Work out the finished part from the listing and answer in its coordinate system (mm). Face numbers are marked on the shaded views. A direction names the side the tool comes from. Give positions to 0.01 mm unless a question says otherwise; leave off trailing zeros. Loops run counter-clockwise (first coordinate to the right, second up) from the corner with the lowest first, then second, coordinate; pieces in that order, holes last. Notation, with made-up numbers: M 32,70.25 L 61,70.25 A21 ccw 61,80.25 Z; hole C 45,9 d1. An arc over 180 degrees is marked long. Use a Markdown table: item, result.
```python
from build123d import *

# Parameters (mm, degrees)
F1_DEPTH = 100
F2_R     = 40
F3_DEPTH = 25
F4_R     = 5
F5_DEPTH = 50


with BuildPart() as f1:
    # F0 (on Front) → F1 (new body)
    with BuildSketch(Plane.XZ):
        with BuildLine():
            Line((-58.053203, 88.663405), (-160.553203, 88.663405))
            ThreePointArc((-160.553203, 88.663405), (-164.088737, 87.198939), (-165.553203, 83.663405))
            Line((-165.553203, 83.663405), (-165.553203, -56.336595))
            ThreePointArc((-165.553203, -56.336595), (-164.088737, -59.872129), (-160.553203, -61.336595))
            Line((-160.553203, -61.336595), (129.446797, -61.336595))
            ThreePointArc((129.446797, -61.336595), (132.98233, -59.872129), (134.446797, -56.336595))
            Line((134.446797, -56.336595), (134.446797, 83.663405))
            ThreePointArc((134.446797, 83.663405), (132.98233, 87.198939), (129.446797, 88.663405))
            Line((129.446797, 88.663405), (26.946797, 88.663405))
            ThreePointArc((26.946797, 88.663405), (23.411263, 87.198939), (21.946797, 83.663405))
            Line((21.946797, 83.663405), (21.946797, 43.663405))
            ThreePointArc((21.946797, 43.663405), (20.48233, 40.127871), (16.946797, 38.663405))
            Line((16.946797, 38.663405), (-48.053203, 38.663405))
            ThreePointArc((-48.053203, 38.663405), (-51.588737, 40.127871), (-53.053203, 43.663405))
            Line((-53.053203, 43.663405), (-53.053203, 83.663405))
            ThreePointArc((-53.053203, 83.663405), (-54.51767, 87.198939), (-58.053203, 88.663405))
        make_face()
    extrude(amount=F1_DEPTH)

    # F2 (on face) → F3 (cut)
    with BuildSketch(Plane.XZ.offset(100)):
        with Locations((-115.553203, -6.336595)):
            Circle(F2_R)
        with Locations((84.446797, -6.336595)):
            Circle(F2_R)
    extrude(amount=-F3_DEPTH, mode=Mode.SUBTRACT)

    # F4 (on face) → F5 (cut)
    with BuildSketch(Plane.XY.offset(38.663405)):
        with Locations((-15.553203, -82.352199)):
            Circle(F4_R)
    extrude(amount=-F5_DEPTH, mode=Mode.SUBTRACT)


solid = f1.part
```
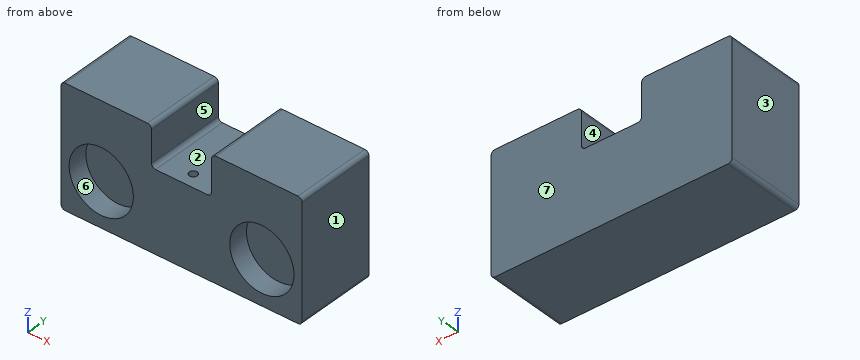
(1) A cutting plane is placed at A-A (z = 70.5). Write down the section's boundary in (x, y).
Entries:
| item | result |
|---|---|
| outline | M -165.55,-100 L -53.05,-100 L -53.05,0 L -165.55,0 Z; M 21.95,-100 L 134.45,-100 L 134.45,0 L 21.95,0 Z |
(2) Given P1, Ø24, axis at x = -134, z = -26, coming from the -Y side; P2, Ø3, axis at x = -15.5, y = -83.5, coming from the +Z side; P3, Ø3, axis at x = -109.5, z = -42.5, coming from the +Y side, each flat-ended and moving along its own axis, determine where each tip first touches the part or whether it passes through.
Entries:
| item | result |
|---|---|
| P1 | stops at y = -75 |
| P2 | stops at z = -11.34 |
| P3 | stops at y = 0 |
(3) Which of the six approach directions +Z, -Z, +X, -X, +Y, -Y give full straight-line access (tool end or side, diameter ignored) to the marked faces 5, 6 and 7?
Entries:
| item | result |
|---|---|
| face 5 | +Z, +Y, -Y |
| face 6 | -Y |
| face 7 | +Z, -Z, +X, -X, +Y |
(4) A cutting plane is placed at D-D (z = -43). Write down the section's boundary in (x, y).
Entries:
| item | result |
|---|---|
| outline | M -165.55,-100 L -131.55,-100 L -131.55,-75 L -99.56,-75 L -99.56,-100 L 68.45,-100 L 68.45,-75 L 100.44,-75 L 100.44,-100 L 134.45,-100 L 134.45,0 L -165.55,0 Z |
(5) A cutting plane is placed at B-B (y = -70.5). Write down the section's boundary in (x, z).
Entries:
| item | result |
|---|---|
| outline | M -165.55,-56.34 A5 ccw -160.55,-61.34 L 129.45,-61.34 A5 ccw 134.45,-56.34 L 134.45,83.66 A5 ccw 129.45,88.66 L 26.95,88.66 A5 ccw 21.95,83.66 L 21.95,43.66 A5 cw 16.95,38.66 L -48.05,38.66 A5 cw -53.05,43.66 L -53.05,83.66 A5 ccw -58.05,88.66 L -160.55,88.66 A5 ccw -165.55,83.66 Z |
(6) The mould has two halves that part along X. Classify the marked faces 1, 2, 3 and 4: released by +X, released by -X, zero draft, split by the parting line, or undercut.
Entries:
| item | result |
|---|---|
| face 1 | released by +X |
| face 2 | undercut |
| face 3 | released by -X |
| face 4 | undercut |
(7) Consider probe 1 along X at (y, z) = (-5, 53.5); probe 2 along X at (y, z) = (-75.5, -6); probe 3 along X at (y, z) = (-93.5, -22.5). Determine where each line is inside the solid, lowest interval first. Write a range as [from, to].
Entries:
| item | result |
|---|---|
| probe 1 | x = [-165.55, -53.05], [21.95, 134.45] |
| probe 2 | x = [-165.55, -155.55], [-75.55, 44.45], [124.45, 134.45] |
| probe 3 | x = [-165.55, -152.14], [-78.96, 47.86], [121.04, 134.45] |
(8) A cutting plane is placed at C-C (x = -126). Write down the section's boundary in (y, z).
Entries:
| item | result |
|---|---|
| outline | M -100,-61.34 L 0,-61.34 L 0,88.66 L -100,88.66 L -100,32.28 L -75,32.28 L -75,-44.95 L -100,-44.95 Z |
